from build123d import *

# Parameters (mm, degrees)
SKETCH1_R           = 6.3373
BOSS_EXTRUDE1_DEPTH = 0.79375


with BuildPart() as part:
    # Sketch1 → Boss-Extrude1 (new, symmetric)
    with BuildSketch(Plane.XY):
        with BuildLine():
            Line((5.08, -7.9375), (-5.08, -7.9375))
            ThreePointArc((-5.08, -7.9375), (-13.0175, 0), (-5.08, 7.9375))
            Line((-5.08, 7.9375), (5.08, 7.9375))
            ThreePointArc((5.08, 7.9375), (13.0175, 0), (5.08, -7.9375))
        make_face()
        Circle(SKETCH1_R, mode=Mode.SUBTRACT)
    extrude(amount=BOSS_EXTRUDE1_DEPTH, both=True)


solid = part.part
Verification items for the finished model (mm, model axes). Give positions to 0.01 mm unless a question says otherwise; leave off trailing zeros. Write each loop counter-clockwise with the first axis right and the second up, starting at its lowest first coordinate (ties: lowest second). Pieces come first, ordered by that corner, then holes. Notation, with made-up numbers: M 74,48.5 L 124,48.5 A9 cw 124,64.5 Z; hole C 53.25,3 d5. An arc over 180 degrees is marked long. Put each result on its own line as item: value. Start each with the question number.
1. Section check D-D (x = -6.75). Record the cut outline in (y, z).
2. Section check B-B (y = 3.5). Record the cut outline in (x, z), and give its area (3 significant figures).
3. Go/stop test with a flat-tipped pin: pin 1 Ø5 at (x, y) = (1.5, 1) entering from +Z. Record where the tip stops, or that it passes through.
4. Section check A-A (x = 0). Record the cut outline in (y, z).
5. Draft check along Y on faces 1 (the face through (0, 7.938, 0)), 2 (the face through (-5.029, -3.856, -0.011)), 3 (the face through (-6, -3, 0.794)). Enter one of: +Y half, -Y half, draft (parallel to the pull), parting line (faces both ways), or undercut.
6. Scan lines: line 1 along Y through (x, z) = (0, -0.3); line 2 along X through (y, z) = (-0.25, 0.3); line 3 along Y through (x, z) = (4.5, -0.6). Record each from-to range of solid material in increasing order. Write a range as [from, to].
7. Section check C-C (z = -0.3). Record the cut outline in (x, y) (1 decimal).
Answer list:
1. outline: M -7.76,-0.79 L 7.76,-0.79 L 7.76,0.79 L -7.76,0.79 Z
2. outline: M -12.2,-0.79 L -5.28,-0.79 L -5.28,0.79 L -12.2,0.79 Z; M 5.28,-0.79 L 12.2,-0.79 L 12.2,0.79 L 5.28,0.79 Z
2. area: 22.0 mm2
3. pin 1: through
4. outline: M -7.94,-0.79 L -6.34,-0.79 L -6.34,0.79 L -7.94,0.79 Z; M 6.34,-0.79 L 7.94,-0.79 L 7.94,0.79 L 6.34,0.79 Z
5. face 1: +Y half
5. face 2: undercut
5. face 3: draft
6. line 1: [-7.94, -6.34], [6.34, 7.94]
6. line 2: [-13.01, -6.33], [6.33, 13.01]
6. line 3: [-7.94, -4.46], [4.46, 7.94]
7. outline: M -5.1,-7.9 L 5.1,-7.9 A7.9 ccw 5.1,7.9 L -5.1,7.9 A7.9 ccw Z; hole C 0,0 d12.7
